```python
from build123d import *

# Parameters (mm, degrees)
F0_W     = 90.503112
F0_H     = 48.822132
F1_DEPTH = 76.2
F2_W     = 73.306068
F2_H     = 57.129182
F3_DEPTH = 76.2
F4_R     = 10.024428
F5_DEPTH = 101.6
F6_W     = 42.263934
F6_H     = 15.593934
F7_DEPTH = 101.6


with BuildPart() as f1:
    # F0 (on Front) → F1 (new body)
    with BuildSketch(Plane.XZ):
        Rectangle(F0_W, F0_H)
    extrude(amount=F1_DEPTH)

    # F2 (on face) → F3 (cut)
    with BuildSketch(Plane(origin=(0, 0, -24.411066), x_dir=(1, 0, 0), z_dir=(0, 0, -1))):
        with Locations((0, 40.005002)):
            Rectangle(F2_W, F2_H)
    extrude(amount=-F3_DEPTH, mode=Mode.SUBTRACT)

    # F4 (on face) → F5 (cut)
    with BuildSketch(Plane(origin=(-45.251556, 0, 0), x_dir=(0, -1, 0), z_dir=(-1, 0, 0))):
        with Locations((42.045325, 0)):
            Circle(F4_R)
    extrude(amount=-F5_DEPTH, mode=Mode.SUBTRACT)

    # F6 (on face) → F7 (cut)
    with BuildSketch(Plane.XZ.offset(76.2)):
        with Locations((0.801557, 16.614099)):
            Rectangle(F6_W, F6_H)
    extrude(amount=-F7_DEPTH, mode=Mode.SUBTRACT)


solid = f1.part
```
Input: part model. Units: mm. Frame: model coordinates. A direction names the side the tool comes from. Round coordinates to 2 decimals unless told otherwise and drop trailing zeros. Order: outer loops, then holes, each group sorted by start corner. A loop starts at its lowest first (then second) coordinate and runs counter-clockwise, first axis right, second up. Notation, with made-up numbers: (79.5, -17) - (110.5, -17) arc R22 ccw to (110.5, 19) - close; hole circle Ø9 at (5.5, -4.75). An arc over 180 degrees is marked (long way). One line per question, with ' | ' between items. Start each with the question number.
1) Contact query for flat-ended pins moving along their axis: P1, Ø3.5, axis at x = -7, y = -6, coming from the +Z side; P2, Ø8, axis at x = 24.5, z = 16.5, coming from the +Y side; P3, Ø5, axis at x = 10.5, z = 12.5, coming from the +Y side. Output: stop coordinate, or through.
2) Cut plane A-A, the plane z = 0. Return the cut outline in (x, y), then the cut area to 3 significant figures.
3) Pull-direction query (Z, two-part tool) for faces 1 (the flat face through (21.934, -6, 17)), 2 (the flat face through (-39, -38, 24.411)), 3 (the cylindrical face through (40.892, -34.657, 6.775)); classes: +Z half, -Z half, draft (parallel to the pull), parting line (faces both ways), or undercut.
4) Cut plane C-C, the plane x = -13. Return the cut outline in (y, z).
5) Ray query, probe 1 along Y at (x, z) = (-18, -4.5); probe 2 along X at (y, z) = (-15.5, -14.5); probe 3 along Z at (x, y) = (-17, -10). Return the intervals inside material, ascending.
6) Cut plane D-D, the plane y = -36. Return the cut outline in (x, z), then the cut area to 3 significant figures.
7) Set-up query: faces 4 (the flat face through (21.934, -72, 17)), 5 (the flat face through (-45.252, -29, 0)), 6 (the flat face through (-1, -11.44, -6)). Return all of +Z, -Z, +X, -X, +Y, -Y with unobstructed straight access to the full face (end or side cutting, diameter ignored); none if empty.
8) Cut plane B-B, the plane y = -59. Return the cut outline in (x, z), then the cut area to 3 significant figures.
Worked out:
1) P1: stops at z = 8.82 | P2: stops at y = 0 | P3: passes through
2) outline: (-45.25, -76.2) - (45.25, -76.2) - (45.25, -52.07) - (36.65, -52.07) - (36.65, -68.57) - (-36.65, -68.57) - (-36.65, -52.07) - (-45.25, -52.07) - close; (-45.25, -32.02) - (-36.65, -32.02) - (-36.65, -11.44) - (36.65, -11.44) - (36.65, -32.02) - (45.25, -32.02) - (45.25, 0) - (-45.25, 0) - close | area: 2,360 mm^2
3) face 1: draft | face 2: +Z half | face 3: undercut
4) outline: (-76.2, -24.41) - (-68.57, -24.41) - (-68.57, 8.82) - (-76.2, 8.82) - close; (-11.44, -24.41) - (0, -24.41) - (0, 8.82) - (-11.44, 8.82) - close
5) probe 1: y = -76.2 to -68.57, -11.44 to 0 | probe 2: x = -45.25 to -36.65, 36.65 to 45.25 | probe 3: z = -24.41 to 8.82
6) outline: (-45.25, -24.41) - (-36.65, -24.41) - (-36.65, -8) - (-45.25, -8) - close; (-45.25, 8) - (-36.65, 8) - (-36.65, 24.41) - (-45.25, 24.41) - close; (36.65, -24.41) - (45.25, -24.41) - (45.25, -8) - (36.65, -8) - close; (36.65, 8) - (45.25, 8) - (45.25, 24.41) - (36.65, 24.41) - close | area: 565 mm^2
7) face 4: +Z, +Y, -Y | face 5: +Z, -Z, -X, +Y, -Y | face 6: +Z, -Z
8) outline: (-45.25, -24.41) - (-36.65, -24.41) - (-36.65, 24.41) - (-45.25, 24.41) - close; (36.65, -24.41) - (45.25, -24.41) - (45.25, 24.41) - (36.65, 24.41) - close | area: 840 mm^2
